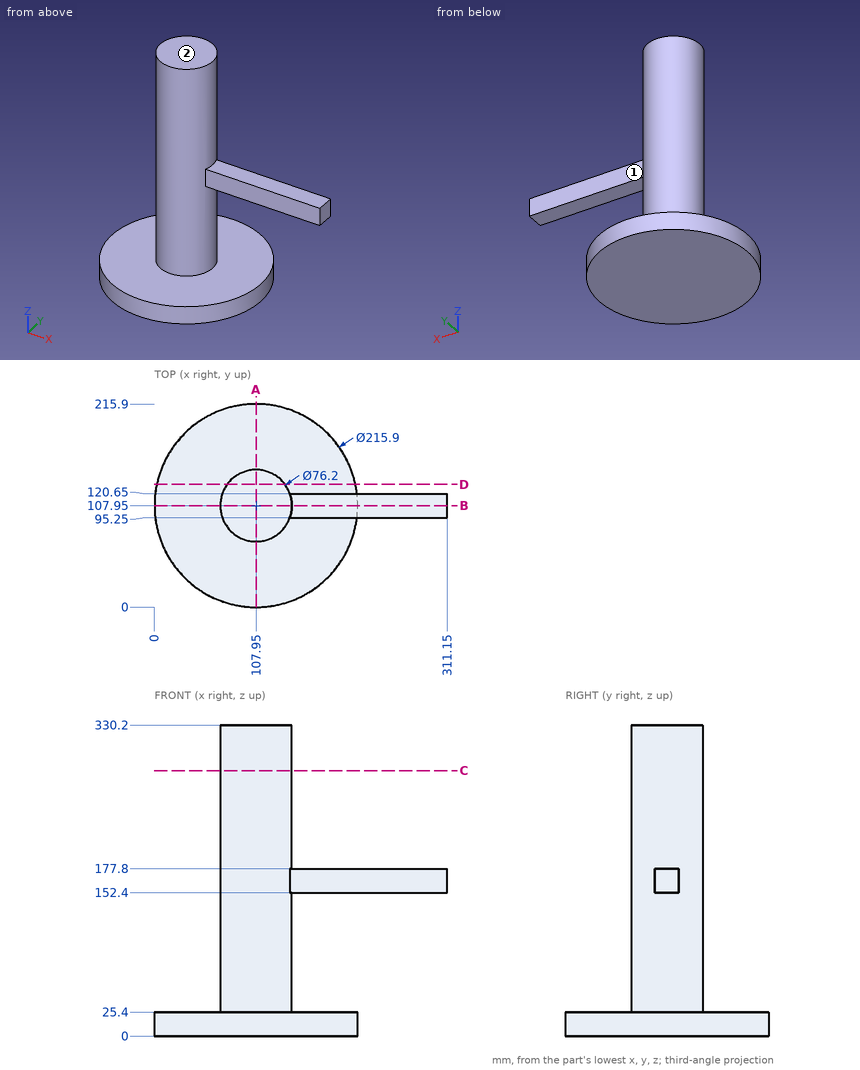
Study the drawing (mm; zero at the part's minimum x, y, z) and answer. A direction names the side the tool comes from. Give positions to 0.01 mm unless a question says otherwise; leave off trailing zeros. Order: outer loops, then holes, each group sorted by start corner. A loop starts at its lowest first (then second) coordinate and runs counter-clockwise, first axis right, second up. Notation, with made-up numbers: (38, 57.5) - (97, 57.5) arc R26 cw to (97, 79.5) - close; hole circle Ø8 at (51.25, 69.5). An arc over 180 degrees is marked (long way). Use one line per item in the form item = value. Start each with the question number.
(1) Consider line 1 (Z direction, x = 196, y = 66); line 2 (Y direction, x = 276.5, z = 171.5); line 3 (Z direction, x = 182.5, y = 101.5). Determine where each line is inside the solid, lowest interval first. Write a range as from..to.
(2) Flat-ended cylindrical pins translate along their axes: pin 1 Ø1 at (x, z) = (87, 259) entering from +Y; pin 2 Ø10 at (x, y) = (41, 119) entering from -Z; pin 3 Ø12.5 at (x, y) = (265.5, 102) entering from +Z; pin 4 Ø10 at (x, z) = (92, 93.5) entering from -Y. Find the tip coordinate at first contact, or state that the pin passes through.
(3) A cutting plane is placed at A-A, the plane x = 107.95. Write down the section's boundary in (y, z), then the cut area to 3 significant figures.
(4) A cutting plane is placed at B-B, the plane y = 107.95. Write down the section's boundary in (x, z), then the cut area to 3 significant figures.
(5) For the marked faces 1 and 2, determine the directions among +Z, -Z, +X, -X, +Y, -Y from which every point of the face is accessible in a straight line to the end or side of a thin tool.
(6) A cutting plane is placed at C-C, the plane z = 282. Write down the section's boundary in (x, y), then the cut area to 3 significant figures.
(7) A cutting plane is placed at D-D, the plane y = 130.5. Write down the section's boundary in (x, z), then the cut area to 3 significant figures.
Ans:
q1.line_1 = 0..25.4
q1.line_2 = 95.25..120.65
q1.line_3 = 0..25.4, 152.4..177.8
q2.pin_1 = 140.1
q2.pin_2 = 0
q2.pin_3 = 177.8
q2.pin_4 = 71.46
q3.outline = (0, 0) - (215.9, 0) - (215.9, 25.4) - (146.05, 25.4) - (146.05, 330.2) - (69.85, 330.2) - (69.85, 25.4) - (0, 25.4) - close
q3.area = 28,700 mm^2
q4.outline = (0, 0) - (215.9, 0) - (215.9, 25.4) - (146.05, 25.4) - (146.05, 152.4) - (311.15, 152.4) - (311.15, 177.8) - (146.05, 177.8) - (146.05, 330.2) - (69.85, 330.2) - (69.85, 25.4) - (0, 25.4) - close
q4.area = 32,900 mm^2
q5.face_1 = +Z, +X, +Y
q5.face_2 = +Z, +X, -X, +Y, -Y
q6.outline = circle Ø76.2 at (107.95, 107.95)
q6.area = 4,560 mm^2
q7.outline = (2.38, 0) - (213.52, 0) - (213.52, 25.4) - (138.66, 25.4) - (138.66, 330.2) - (77.24, 330.2) - (77.24, 25.4) - (2.38, 25.4) - close
q7.area = 24,100 mm^2
